For this review, take the finished solid that the model builds, in its own axes (mm). Give positions to 0.01 mm unless a question says otherwise; leave off trailing zeros. Loops run counter-clockwise (first coordinate to the right, second up) from the corner with the lowest first, then second, coordinate; pieces in that order, holes last. Notation, with made-up numbers: (39, -8.75) - (74, -8.75) arc R35 cw to (74, 26.25) - close; hole circle Ø5 at (71.25, 26). An arc over 180 degrees is marked (long way). Answer as CSV lines item,"result".
Autodesk Inventor part; units mm, degrees
ref_plane "YZ Plane" through (0, 0, 0) normal (1, 0, 0) x (0, 1, 0)
ref_plane "XZ Plane" through (0, 0, 0) normal (0, 1, 0) x (-1, 0, 0)
ref_plane "XY Plane" through (0, 0, 0) normal (0, 0, 1) x (1, 0, 0)
sketch "Sketch1" plane through (0, 0, 0) normal (0, 0, 1) x (1, 0, 0)
  line L0 (-20.32, 26.67) -> (20.32, 26.67)
  line L1 (20.32, 26.67) -> (20.32, -26.67)
  line L2 (20.32, -26.67) -> (-20.32, -26.67)
  line L3 (-20.32, -26.67) -> (-20.32, 26.67)
  point P0 (0, 0)
  point P1 (20.32, 0)
  point P2 (0, 26.67)
  dimension "d0" = 40.64
  dimension "d1" = 53.34
extrude "Extrusion1" add sketch "Sketch1" along normal blind 25
sketch "Sketch2" plane through (0, 0, 25) normal (0, 0, 1) x (1, 0, 0)
  circle A0 centre (0, 6.0325) radius 7.5
  line L0 (20.32, 26.67) -> (-20.32, 26.67)
  circle A1 centre (0, -14.2875) radius 3.175
  line L1 (0, 6.0325) -> (44.8131, 6.0325) construction
  line L2 (0, 6.0325) -> (0, 52.3228) construction
  circle A2 centre (15.5, 21.5325) radius 1.5875
  circle A3 centre (-15.5, 21.5325) radius 1.5875
  circle A4 centre (15.5, -9.4675) radius 1.5875
  circle A5 centre (-15.5, -9.4675) radius 1.5875
  point P0 (0, 0)
  dimension "d4" = 20.6375
  dimension "d5" = 15
  dimension "d8" = 6.35
  dimension "d9" = 20.32
  dimension "d11" = 3.175
  dimension "d12" = 15.5
  dimension "d13" = 15.5
extrude "Extrusion2" cut sketch "Sketch2" against normal up to surface (25 mm away)
sketch "Sketch3" plane through (-20.32, 26.67, 0) normal (0, 1, 0) x (1, 0, 0)
  line L0 (0, 0) -> (0, -25)
  line L1 (0, -25) -> (40.64, -25)
  line L2 (0, 0) -> (40.64, 0)
  line L3 (40.64, 0) -> (40.64, -25)
  line L4 (40.64, -25) -> (0, -25)
  line L5 (0, -25) -> (0, 0)
  point P0 (20.32, 0)
extrude "Extrusion3" cut sketch "Sketch3" against normal blind 1.27
fillet "Fillet1" radius 1.6002 4 edges at (20.32, 25.4, 12.5) (-20.32, 25.4, 12.5) (20.32, -26.67, 12.5) (-20.32, -26.67, 12.5)
properties part number "Motor Brace"
1) Consider section A-A on x = -15.5. Write out the cut boundary in (y, z) (3 decimals).
From the geometry:
outline,"(-26.67, 0) - (-11.055, 0) - (-11.055, 25) - (-26.67, 25) - close; (-7.88, 0) - (19.945, 0) - (19.945, 25) - (-7.88, 25) - close; (23.12, 0) - (25.4, 0) - (25.4, 25) - (23.12, 25) - close"
2) Draft analysis for pull direction Y (two halves, no side actions). For faces 1 (the cylindrical face through (-19.84, 24.94, 12.68)), 2 (the cylindrical face through (-1.63, -1.29, 12.68)), 3 (the flat face through (0, -26.67, 12)), state which applies: pulls with the +Y half, pulls with the -Y half, needs draft (parallel to the pull), parting line crosses it, or undercut.
From the geometry:
face 1,"pulls with the +Y half"
face 2,"undercut"
face 3,"pulls with the -Y half"
3) Consider section B-B on y = 5. Write out the cut boundary in (x, z), and give its area (3 significant figures).
From the geometry:
outline,"(-20.32, 0) - (-7.43, 0) - (-7.43, 25) - (-20.32, 25) - close; (7.43, 0) - (20.32, 0) - (20.32, 25) - (7.43, 25) - close"
area,"645 mm^2"
4) Insertion check: P1, Ø3, axis at x = -15.5, y = 21.53, coming from the -Z side (1 decimal); P2, Ø2, axis at x = -15, y = 0, coming from the -Z side. Each pin has a flat end and moves straight along its axis. Give the tip position at first contact, or say it passes through.
From the geometry:
P1,"passes through"
P2,"stops at z = 0"
5) Wall thickness on line 1 (Y direction, x = 0, z = 17.25); line 2 (Y direction, x = 15.5, z = 18.5) (3 decimals); line 3 (X direction, y = 1.5, z = 9.5): over which ranges is each line inside the solid? List them lowest first. Write a range as from..to.
From the geometry:
line 1,"y = -26.67..-17.46, -11.11..-1.47, 13.53..25.4"
line 2,"y = -26.67..-11.055, -7.88..19.945, 23.12..25.4"
line 3,"x = -20.32..-5.98, 5.98..20.32"
6) Consider section D-D on z = 16. Count the separate pieces of the cut face and the enclosed holes in it, and give its area (3 significant figures).
From the geometry:
separate pieces,"1"
enclosed holes,"6"
area,"1,870 mm^2"
7) Consider section C-C on x = 0. Write out the cut boundary in (y, z).
From the geometry:
outline,"(-26.67, 0) - (-17.46, 0) - (-17.46, 25) - (-26.67, 25) - close; (-11.11, 0) - (-1.47, 0) - (-1.47, 25) - (-11.11, 25) - close; (13.53, 0) - (25.4, 0) - (25.4, 25) - (13.53, 25) - close"
